```python
from build123d import *

# Parameters (mm, degrees)
SKETCH1_W           = 5
SKETCH1_H           = 15
BOSS_EXTRUDE1_DEPTH = 5
SKETCH2_W           = 5
SKETCH2_H           = 2
BOSS_EXTRUDE2_DEPTH = 10
SKETCH3_R           = 1.05
CUT_EXTRUDE1_DEPTH  = 10


with BuildPart() as part:
    # Sketch1 → Boss-Extrude1 (new body)
    with BuildSketch(Plane.XY):
        with Locations((2.5, 7.5)):
            Rectangle(SKETCH1_W, SKETCH1_H)
    extrude(amount=BOSS_EXTRUDE1_DEPTH)

    # Sketch2 → Boss-Extrude2 (add)
    with BuildSketch(Plane.XY.offset(5)):
        with Locations((2.5, 1)):
            Rectangle(SKETCH2_W, SKETCH2_H)
    extrude(amount=BOSS_EXTRUDE2_DEPTH)

    # Sketch3 → Cut-Extrude1 (cut)
    with BuildSketch(Plane.XY.offset(5)):
        with Locations((2.5, 11.4)):
            Circle(SKETCH3_R)
    extrude(amount=-CUT_EXTRUDE1_DEPTH, mode=Mode.SUBTRACT)


solid = part.part
```
Source: CAD feature listing. Evaluate the final solid. Frame: model axes, mm. A direction names the side the tool comes from. Give positions to 0.01 mm unless a question says otherwise; leave off trailing zeros. Order: outer loops, then holes, each group sorted by start corner. A loop starts at its lowest first (then second) coordinate and runs counter-clockwise, first axis right, second up.
(1) Section query B-B (x = 2.5). Return the cut outline in (y, z).
(2) Section query D-D (x = 1). Return the cut outline in (y, z), plus the area to 3 significant figures.
(3) Contact query for flat-ended pins moving along their axis: P1, Ø2, axis at x = 4.5, z = 8, coming from the +Y side; P2, Ø1.9, axis at x = 2.5, y = 11.4, coming from the +Z side; P3, Ø2.5, axis at x = 2.5, y = 8.5, coming from the +Z side. Output: stop coordinate, or through.
(4) Pull-direction query (Y, two-part tool) for faces 1 (the face through (2.272, 10.375, 2.535)), 2 (the face through (2, 0, 7)), 3 (the face through (2, 9, 5)); classes: +Y half, -Y half, draft (parallel to the pull), parting line (faces both ways), or undercut.
(5) Material intervals for line 1 along Y through (x, z) = (2.5, 1.8); line 2 along Z through (x, y) = (1.25, 8.5); line 3 along Y through (x, z) = (2.55, 7), sorted ascending.
(6) Section query A-A (y = 11.4). Return the cut outline in (x, z).
(7) Access query for faces 4 (the face through (2, 1, 15)), 5 (the face through (2, 2, 10)). Directions: +Z, -Z, +X, -X, +Y, -Y. A direction counts if a zero-diameter tool reaches every point of the face in a straight line with its end or side. Return the directions, or none.
(8) Section query C-C (z = 4.75). Return the cut outline in (x, y).
Outcome:
1. outline: (0, 0) - (10.35, 0) - (10.35, 5) - (2, 5) - (2, 15) - (0, 15) - close; (12.45, 0) - (15, 0) - (15, 5) - (12.45, 5) - close
2. outline: (0, 0) - (15, 0) - (15, 5) - (2, 5) - (2, 15) - (0, 15) - close
2. area: 95.0 mm2
3. P1: stops at y = 2
3. P2: passes through
3. P3: stops at z = 5
4. face 1: undercut
4. face 2: -Y half
4. face 3: draft
5. line 1: y = 0 to 10.35, 12.45 to 15
5. line 2: z = 0 to 5
5. line 3: y = 0 to 2
6. outline: (0, 0) - (1.45, 0) - (1.45, 5) - (0, 5) - close; (3.55, 0) - (5, 0) - (5, 5) - (3.55, 5) - close
7. face 4: +Z, +X, -X, +Y, -Y
7. face 5: +Z, +X, -X, +Y
8. outline: (0, 0) - (5, 0) - (5, 15) - (0, 15) - close; hole circle Ø2.1 at (2.5, 11.4)
